Here's how the part is built. I have some questions about the finished solid (model axes, mm). A direction names the side the tool comes from. Coordinates: 2 decimals unless noted, no trailing zeros. Loops run counter-clockwise (first coordinate to the right, second up) from the corner with the lowest first, then second, coordinate; pieces in that order, holes last.
from build123d import *

# Parameters (mm, degrees)
BASE_EXTRUDE_START                = -77
BASE_EXTRUDE_DEPTH                = 77
SKETCH2_R                         = 8
CUT_EXTRUDE1_DEPTH                = 75.7
SKETCH4_R                         = 8
BOSS_EXTRUDE1_DEPTH               = 10
CUT_EXTRUDE3_REACH                = 82.789
SKETCH19_R                        = 4
F_1_4_20_TAPPED_HOLE1_D           = 5.1054
F_1_4_20_TAPPED_HOLE1_DEPTH       = 26.162
F_1_4_20_TAPPED_HOLE1_CBORE_D     = 6.35
F_1_4_20_TAPPED_HOLE1_CBORE_DEPTH = 19.812
F_1_4_20_TAPPED_HOLE1_TIP         = 1.533816902
F_8_32_TAPPED_HOLE1_D             = 3.4544
F_8_32_TAPPED_HOLE1_DEPTH         = 10.8204
F_8_32_TAPPED_HOLE1_CBORE_D       = 4.1656
F_8_32_TAPPED_HOLE1_CBORE_DEPTH   = 6.858
F_8_32_TAPPED_HOLE1_TIP           = 1.037806461
HOLE1_D                           = 5
HOLE1_DEPTH                       = 4
CUT_EXTRUDE4_DEPTH                = 4
F_10_32_TAPPED_HOLE1_D            = 4.0386
F_10_32_TAPPED_HOLE1_DEPTH        = 13.6144
F_10_32_TAPPED_HOLE1_CBORE_D      = 4.826
F_10_32_TAPPED_HOLE1_CBORE_DEPTH  = 9.652
F_10_32_TAPPED_HOLE1_TIP          = 1.213317848
SKETCH30_W                        = 35
SKETCH30_H                        = 37
BOSS_EXTRUDE2_DEPTH               = 10
BOSS_EXTRUDE3_DEPTH               = 3
SKETCH35_R                        = 2.5
BOSS_EXTRUDE5_DEPTH               = 3
CHAMFER2_SIZE                     = 0.5
BOSS_EXTRUDE6_DEPTH               = 10
BOSS_EXTRUDE7_DEPTH               = 3
CUT_EXTRUDE7_REACH                = 109.959
SKETCH38_R                        = 6
CUT_EXTRUDE8_REACH                = 142.905
SKETCH46_R                        = 6
CHAMFER3_SIZE                     = 1


with BuildPart() as part:
    # Sketch1 → Base-Extrude (new body)
    with BuildSketch(Plane(origin=(0, 0, 51.15), x_dir=(-1, 0, 0), z_dir=(0, 0, 1)).offset(BASE_EXTRUDE_START)):
        with BuildLine():
            Line((27.615, 10.1854), (28.25, 9.5504))
            Line((28.25, 9.5504), (28.25, -9.5504))
            Line((28.25, -9.5504), (27.615, -10.1854))
            Line((27.615, -10.1854), (8.763, -10.1854))
            Line((8.763, -10.1854), (8.128, -9.5504))
            Line((8.128, -9.5504), (-8.128, -9.5504))
            Line((-8.128, -9.5504), (-8.763, -10.1854))
            Line((-8.763, -10.1854), (-27.615, -10.1854))
            Line((-27.615, -10.1854), (-28.25, -9.5504))
            Line((-28.25, -9.5504), (-28.25, -5.4483))
            Line((-28.25, -5.4483), (-27.384444989, -5.4483))
            ThreePointArc((-27.384444989, -5.4483), (-23.801775541, -3.9116), (-27.384444989, -2.3749))
            Line((-27.384444989, -2.3749), (-28.25, -2.3749))
            Line((-28.25, -2.3749), (-28.25, 2.3749))
            Line((-28.25, 2.3749), (-27.384444989, 2.3749))
            ThreePointArc((-27.384444989, 2.3749), (-23.801775541, 3.9116), (-27.384444989, 5.4483))
            Line((-27.384444989, 5.4483), (-28.25, 5.4483))
            Line((-28.25, 5.4483), (-28.25, 9.5504))
            Line((-28.25, 9.5504), (-27.615, 10.1854))
            Line((-27.615, 10.1854), (-8.763, 10.1854))
            Line((-8.763, 10.1854), (-8.128, 9.5504))
            Line((-8.128, 9.5504), (8.128, 9.5504))
            Line((8.128, 9.5504), (8.763, 10.1854))
            Line((8.763, 10.1854), (27.615, 10.1854))
        make_face()
    extrude(amount=BASE_EXTRUDE_DEPTH)

    # Sketch2 → Cut-Extrude1 (cut)
    with BuildSketch(Plane(origin=(0, 0, 51.15), x_dir=(-1, 0, 0), z_dir=(0, 0, -1))):
        with Locations(Location((-14.859, 0, 0), (0, 0, 180))):
            Circle(SKETCH2_R)
        with Locations(Location((13.5128, 0, 0), (0, 0, 180))):
            Circle(SKETCH2_R)
    extrude(amount=CUT_EXTRUDE1_DEPTH, mode=Mode.SUBTRACT)

    # Sketch4 → Boss-Extrude1 (add)
    with BuildSketch(Plane.XY.offset(49.15)):
        with Locations((14.859, 0)):
            Circle(SKETCH4_R)
        with Locations((-13.5128, 0)):
            Circle(SKETCH4_R)
    extrude(amount=-BOSS_EXTRUDE1_DEPTH)

    # Sketch19 → Cut-Extrude3 (cut, up to next)
    with BuildSketch(Plane.XY.offset(49.15), mode=Mode.PRIVATE) as cut_extrude3_sk1:
        with Locations((14.859, 0)):
            Circle(SKETCH19_R)
    cut_extrude3_tool1 = extrude(cut_extrude3_sk1.sketch, amount=-CUT_EXTRUDE3_REACH, mode=Mode.PRIVATE) & part.part
    # Sketch19 → Cut-Extrude3 (cut, up to next)
    with BuildSketch(Plane.XY.offset(49.15), mode=Mode.PRIVATE) as cut_extrude3_sk2:
        with Locations((-13.5128, 0)):
            Circle(SKETCH19_R)
    cut_extrude3_tool2 = extrude(cut_extrude3_sk2.sketch, amount=-CUT_EXTRUDE3_REACH, mode=Mode.PRIVATE) & part.part
    add(cut_extrude3_tool1.solids().sort_by_distance((14.859, 0, 49.15))[0], mode=Mode.SUBTRACT)
    add(cut_extrude3_tool2.solids().sort_by_distance((-13.5128, 0, 49.15))[0], mode=Mode.SUBTRACT)

    # 1/4-20 Tapped Hole1
    with Locations(Plane.XZ.offset(9.5504)):
        with Locations((0, 26.15), (0, -3.85)):
            CounterBoreHole(F_1_4_20_TAPPED_HOLE1_D / 2, F_1_4_20_TAPPED_HOLE1_CBORE_D / 2, F_1_4_20_TAPPED_HOLE1_CBORE_DEPTH, depth=F_1_4_20_TAPPED_HOLE1_DEPTH)
            with Locations((0, 0, -(F_1_4_20_TAPPED_HOLE1_DEPTH + F_1_4_20_TAPPED_HOLE1_TIP / 2))):  # 118° drill point
                Cone(0, F_1_4_20_TAPPED_HOLE1_D / 2, F_1_4_20_TAPPED_HOLE1_TIP, mode=Mode.SUBTRACT)

    # #8-32 Tapped Hole1
    with Locations(Plane(origin=(0, 0, -25.85), x_dir=(-1, 0, 0), z_dir=(0, 0, -1))):
        with Locations((25, -5.6854), (25, 5.3146), (-4, -5.6854), (-4, 5.3146)):
            CounterBoreHole(F_8_32_TAPPED_HOLE1_D / 2, F_8_32_TAPPED_HOLE1_CBORE_D / 2, F_8_32_TAPPED_HOLE1_CBORE_DEPTH, depth=F_8_32_TAPPED_HOLE1_DEPTH)
            with Locations((0, 0, -(F_8_32_TAPPED_HOLE1_DEPTH + F_8_32_TAPPED_HOLE1_TIP / 2))):  # 118° drill point
                Cone(0, F_8_32_TAPPED_HOLE1_D / 2, F_8_32_TAPPED_HOLE1_TIP, mode=Mode.SUBTRACT)

    # Hole1
    with Locations(Plane.XZ.offset(10.1854)):
        with Locations((-24, 36.15)):
            Hole(HOLE1_D / 2, depth=HOLE1_DEPTH)

    # Sketch27 → Cut-Extrude4 (cut)
    with BuildSketch(Plane.XZ.offset(10.1854)):
        with BuildLine():
            Line((-26.5, 1.65), (-26.5, 0.65))
            ThreePointArc((-26.5, 0.65), (-24, -1.85), (-21.5, 0.65))
            Line((-21.5, 0.65), (-21.5, 1.65))
            ThreePointArc((-21.5, 1.65), (-24, 4.15), (-26.5, 1.65))
        make_face()
    extrude(amount=-CUT_EXTRUDE4_DEPTH, mode=Mode.SUBTRACT)

    # #10-32 Tapped Hole1
    with Locations(Plane.ZY.offset(28.25)):
        with Locations((30.15, -0.1854), (-21.05, -0.1854)):
            CounterBoreHole(F_10_32_TAPPED_HOLE1_D / 2, F_10_32_TAPPED_HOLE1_CBORE_D / 2, F_10_32_TAPPED_HOLE1_CBORE_DEPTH, depth=F_10_32_TAPPED_HOLE1_DEPTH)
            with Locations((0, 0, -(F_10_32_TAPPED_HOLE1_DEPTH + F_10_32_TAPPED_HOLE1_TIP / 2))):  # 118° drill point
                Cone(0, F_10_32_TAPPED_HOLE1_D / 2, F_10_32_TAPPED_HOLE1_TIP, mode=Mode.SUBTRACT)

    # Sketch30 → Boss-Extrude2 (add)
    with BuildSketch(Plane(origin=(0, 0, -25.85), x_dir=(-1, 0, 0), z_dir=(0, 0, -1))):
        with Locations((10.25, 9.4496)):
            Rectangle(SKETCH30_W, SKETCH30_H)
    extrude(amount=BOSS_EXTRUDE2_DEPTH)

    # Sketch31 → Boss-Extrude3 (add)
    with BuildSketch(Plane(origin=(0, 0, -35.85), x_dir=(-1, 0, 0), z_dir=(0, 0, -1))):
        Polygon((23.832903769, 17.9496), (19.791451884, 24.9496), (11.708548116, 24.9496), (7.667096231, 17.9496), (11.708548116, 10.9496), (19.791451884, 10.9496), align=None)
    extrude(amount=BOSS_EXTRUDE3_DEPTH)

    # Sketch35 → Boss-Extrude5 (add)
    with BuildSketch(Plane(origin=(0, 0, -35.85), x_dir=(-1, 0, 0), z_dir=(0, 0, -1))):
        with Locations((25, 5.3146)):
            Circle(SKETCH35_R)
        with Locations((-4, 5.3146)):
            Circle(SKETCH35_R)
        with Locations((-4, -5.6854)):
            Circle(SKETCH35_R)
        with Locations((25, -5.6854)):
            Circle(SKETCH35_R)
    extrude(amount=BOSS_EXTRUDE5_DEPTH)

    # Chamfer2
    chamfer2_edges = [part.edges().sort_by_distance(p)[0] for p in [
        (-22.5, 5.3146, -38.85),
        (6.5, 5.3146, -38.85),
        (6.5, -5.6854, -38.85),
        (-22.5, -5.6854, -38.85),
    ]]
    chamfer(chamfer2_edges, length=CHAMFER2_SIZE)

    # Sketch36 → Boss-Extrude6 (add)
    with BuildSketch(Plane.XY.offset(41.15)):
        Polygon((-28.75, 29.3146), (-28.75, 8.1854), (-28.25, 8.1854), (-28.25, -8.1854), (-46.25, -8.1854), (-46.25, 29.3146), align=None)
    extrude(amount=BOSS_EXTRUDE6_DEPTH)

    # Sketch37 → Boss-Extrude7 (add)
    with BuildSketch(Plane.XY.offset(51.15)):
        Polygon((-34.208548116, 26.3146), (-42.291451884, 26.3146), (-46.332903769, 19.3146), (-42.291451884, 12.3146), (-34.208548116, 12.3146), (-30.167096231, 19.3146), align=None)
    extrude(amount=BOSS_EXTRUDE7_DEPTH)

    # Sketch38 → Cut-Extrude7 (cut, up to next)
    with BuildSketch(Plane.XY.offset(54.15), mode=Mode.PRIVATE) as cut_extrude7_sk1:
        with Locations((-38.25, 19.3146)):
            Circle(SKETCH38_R)
    cut_extrude7_tool1 = extrude(cut_extrude7_sk1.sketch, amount=-CUT_EXTRUDE7_REACH, mode=Mode.PRIVATE) & part.part
    add(cut_extrude7_tool1.solids().sort_by_distance((-38.25, 19.3146, 54.15))[0], mode=Mode.SUBTRACT)

    # Sketch44 → Boss-Revolve1 (revolve)
    with BuildSketch(Plane(origin=(0, 19.3146, 0), x_dir=(-1, 0, 0), z_dir=(0, 1, 0)), mode=Mode.PRIVATE) as boss_revolve1_sk:
        Polygon((38.25, 90.95), (44.25, 90.95), (44.25, 42.15), (43.25, 41.15), (38.25, 41.15), align=None)
    revolve(boss_revolve1_sk.sketch.rotate(Axis((-38.25, 19.3146, 54.15), (0, 0, -1)), 180), axis=Axis((-38.25, 19.3146, 54.15), (0, 0, -1)))

    # Sketch46 → Cut-Extrude8 (cut, up to next)
    with BuildSketch(Plane(origin=(0, 0, -38.85), x_dir=(-1, 0, 0), z_dir=(0, 0, -1)), mode=Mode.PRIVATE) as cut_extrude8_sk1:
        with Locations((15.75, 17.9496)):
            Circle(SKETCH46_R)
    cut_extrude8_tool1 = extrude(cut_extrude8_sk1.sketch, amount=-CUT_EXTRUDE8_REACH, mode=Mode.PRIVATE) & part.part
    add(cut_extrude8_tool1.solids().sort_by_distance((-15.75, 17.9496, -38.85))[0], mode=Mode.SUBTRACT)

    # Sketch47 → Boss-Revolve2 (revolve)
    with BuildSketch(Plane(origin=(0, 17.9496, 0), x_dir=(-1, 0, 0), z_dir=(0, 1, 0))):
        Polygon((20.75, -25.85), (15.75, -25.85), (15.75, -75.65), (21.75, -75.65), (21.75, -26.85), align=None)
    revolve(axis=Axis((-15.75, 17.9496, -25.85), (0, 0, -1)))

    # Chamfer3
    chamfer3_edges = [part.edges().sort_by_distance(p)[0] for p in [
        (-44.25, 19.3146, 90.95),
        (-9.75, 17.9496, -75.65),
    ]]
    chamfer(chamfer3_edges, length=CHAMFER3_SIZE)


solid = part.part
Q1. For faces 4 (the cylindrical face through (-27, 5.9, -22.5)), 5 (the flat face through (-12, 4, 49.15)), 6 (the flat face through (-10, 10, -35.85)), 7 (the flat face through (-16, 24.95, -37)), 8 (the flat face through (-24, -6.185, 36)), which set-ups out of +Z, -Z, +X, -X, +Y, -Y let a thin tool reach every point of the face, with its end or its side?
Q2. We'd pull the mould along Z, two halves only. Please class faces 1 (the flat face through (17, 4, 49.15)), 2 (the cylindrical face through (-26.726, -5.609, -16.983)), 3 (the flat face through (-28.25, 0, 12)): pulls with the +Z half, pulls with the -Z half, needs draft (parallel to the pull), parting line crosses it, or undercut.
Q3. Suppose I cut it at B-B on x = 0. Write out the boundary of the cut face in (y, z) (3 decimals).
Q4. Please list where these lines run through material, in increasing order: probe 1 along Y at (x, z) = (-25, -24); probe 2 along X at (y, z) = (0, 50.4); probe 3 along X at (y, z) = (0, 26).
Q5. Suppose I cut it at A-A on z = -3.85. State how many separate pieces and enclosed holes the cut face has, and give its area (3 significant figures).
Q6. Will these pins go through, and if not, where does the flat tip stop? P1, Ø5.5, axis at x = 25.92, y = 3.91, coming from the -Z side; P2, Ø17.5, axis at x = -10.5, y = -0.5, coming from the -Z side; P3, Ø0.9, axis at x = -36.5, z = 53, coming from the -Y side; P4, Ø10, axis at y = 17.5, z = 22, coming from the -X side.
Check values:
1. face 4: none
1. face 5: +Z
1. face 6: -Z
1. face 7: -Z, +X, -X, +Y
1. face 8: -Y
2. face 1: pulls with the +Z half
2. face 2: undercut
2. face 3: needs draft
3. outline: (-9.55, -25.85) - (-9.05, -25.85) - (-9.05, -35.85) - (27.95, -35.85) - (27.95, -25.85) - (9.55, -25.85) - (9.55, -7.025) - (-9.55, -7.025) - close; (-9.55, -0.675) - (9.55, -0.675) - (9.55, 22.975) - (-9.55, 22.975) - close; (-9.55, 29.325) - (9.55, 29.325) - (9.55, 51.15) - (-9.55, 51.15) - close
4. probe 1: y = -10.19 to -7.77, -3.6 to 3.23, 7.4 to 10.19
4. probe 2: x = -46.25 to -21.51, -5.51 to 6.86, 22.86 to 28.25
4. probe 3: x = -28.25 to -21.51, -5.51 to -3.17, 3.17 to 6.86, 22.86 to 28.25
5. separate pieces: 2
5. enclosed holes: 2
5. area: 574 mm2
6. P1: stops at z = -25.85
6. P2: stops at z = -35.85
6. P3: stops at y = 12.31
6. P4: passes through
